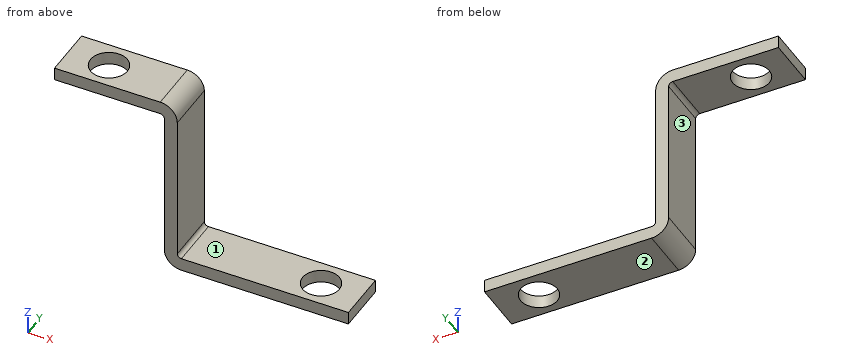
```python
from build123d import *

# Parameters (mm, degrees)
SKETCH1_W                    = 30
SKETCH1_H                    = 12.7
BOSS_EXTRUDE1_DEPTH          = 3.175
EDGE_FLANGE1_STRIP_W         = 14.7
EDGE_FLANGE1_STRIP_H         = 3.175
EDGE_FLANGE1_STRIP_CUT_DEPTH = 12.7
EDGE_FLANGE1_DEPTH           = 12.7
EDGE_FLANGE2_STRIP_W         = 14.7
EDGE_FLANGE2_STRIP_H         = 3.175
EDGE_FLANGE2_STRIP_CUT_DEPTH = 12.7
EDGE_FLANGE2_DEPTH           = 12.7
M8_CLEARANCE_HOLE1_D         = 9


# Sheet-metal steps are written as plain solids
with BuildPart() as part:
    # Sketch1 → Boss-Extrude1 (new body)
    with BuildSketch(Plane.XY):
        with Locations((15, 6.35)):
            Rectangle(SKETCH1_W, SKETCH1_H)
    extrude(amount=BOSS_EXTRUDE1_DEPTH)

    # Edge-Flange1 strip (across the edge) → Edge-Flange1 strip cut (cut)
    with BuildSketch(Plane(origin=(30, 12.7, 0), x_dir=(-1, 0, 0), z_dir=(0, -1, 0))):
        with Locations((-3.175, -1.5875)):
            Rectangle(EDGE_FLANGE1_STRIP_W, EDGE_FLANGE1_STRIP_H)
    extrude(amount=EDGE_FLANGE1_STRIP_CUT_DEPTH, mode=Mode.SUBTRACT)

    # Edge-Flange1 section (across the edge) → Edge-Flange1 (add)
    with BuildSketch(Plane(origin=(30, 12.7, 0), x_dir=(-1, 0, 0), z_dir=(0, -1, 0))):
        with BuildLine():
            Line((0, 1), (0, 41.32))
            Line((0, 41.32), (3.175, 41.32))
            Line((3.175, 41.32), (3.175, 1))
            ThreePointArc((3.175, 1), (3.467893219, 0.292893219), (4.175, 0))
            Line((4.175, 0), (4.175, -3.175))
            ThreePointArc((4.175, -3.175), (1.222829189, -1.952170811), (0, 1))
        make_face()
    extrude(amount=EDGE_FLANGE1_DEPTH)

    # Edge-Flange2 strip (across the edge) → Edge-Flange2 strip cut (cut)
    with BuildSketch(Plane(origin=(30, 0, -41.32), x_dir=(0, 0, 1), z_dir=(0, 1, 0))):
        with Locations((-3.175, -1.5875)):
            Rectangle(EDGE_FLANGE2_STRIP_W, EDGE_FLANGE2_STRIP_H)
    extrude(amount=EDGE_FLANGE2_STRIP_CUT_DEPTH, mode=Mode.SUBTRACT)

    # Edge-Flange2 section (across the edge) → Edge-Flange2 (add)
    with BuildSketch(Plane(origin=(30, 0, -41.32), x_dir=(0, 0, 1), z_dir=(0, 1, 0))):
        with BuildLine():
            Line((0, 1), (0, 41.825))
            Line((0, 41.825), (3.175, 41.825))
            Line((3.175, 41.825), (3.175, 1))
            ThreePointArc((3.175, 1), (3.467893219, 0.292893219), (4.175, 0))
            Line((4.175, 0), (4.175, -3.175))
            ThreePointArc((4.175, -3.175), (1.222829189, -1.952170811), (0, 1))
        make_face()
    extrude(amount=EDGE_FLANGE2_DEPTH)

    # M8 Clearance Hole1 (through all)
    with Locations(Plane(origin=(0, 0, -41.32), x_dir=(-1, 0, 0), z_dir=(0, 0, -1))):
        with Locations((-61.825, 6.35), (-10, 6.35)):
            Hole(M8_CLEARANCE_HOLE1_D / 2)


solid = part.part
```
Check sheet for the modelled part. Datum: model origin and axes. Units: mm. Face numbers are marked on the shaded views. A direction names the side the tool comes from. Give positions to 0.01 mm unless a question says otherwise; leave off trailing zeros. Write each loop counter-clockwise with the first axis right and the second up, starting at its lowest first coordinate (ties: lowest second). Pieces come first, ordered by that corner, then holes. Notation, with made-up numbers: (-3, 60.25) - (16, 60.25) arc R27 cw to (16, 92.25) - close; hole circle Ø9 at (81.5, 42.5). An arc over 180 degrees is marked (long way). Answer as a JSON object with one key per item and string values. Group by question number.
1) Depth check by flat-ended pin: P1, Ø3, axis at x = 28, y = 5.5, coming from the -Z side; P2, Ø6, axis at y = 4, z = -19, coming from the +X side; P3, Ø2, axis at x = 14, y = 6, coming from the -Z side. Enter the tip coordinate at first touch or a pass-through.
2) Sectioned sample at D-D (x = 37). Record the cut outline in (y, z) (3 decimals), then the cut area to 3 significant figures.
3) Sectioned sample at B-B (x = 10). Record the cut outline in (y, z) (3 decimals).
4) Sectioned sample at C-C (z = -7). Record the cut outline in (x, y) (3 decimals).
5) Thickness scan on probe 1 along Y at (x, z) = (10, 1); probe 2 along Z at (x, y) = (5.5, 2.5) (3 decimals); probe 3 along X at (y, z) = (4.75, -6) (3 decimals). Record the ranges inside material, lowest first. Write a range as from..to.
6) Sectioned sample at A-A (y = 6.35). Record the cut outline in (x, z) (3 decimals).
7) Access from +Z, -Z, +X, -X, +Y, -Y to the whole of each face (thin tool, end or side, straight path). Record for the marked faces 1, 2 and 3.
Geometry results:
{
 "1": {"P1": "stops at z = -41.04", "P2": "stops at x = 30", "P3": "stops at z = 0"},
 "2": {"outline": "(0, -41.32) - (12.7, -41.32) - (12.7, -38.145) - (0, -38.145) - close", "area": "40.3 mm^2"},
 "3": {"outline": "(0, 0) - (1.85, 0) - (1.85, 3.175) - (0, 3.175) - close; (10.85, 0) - (12.7, 0) - (12.7, 3.175) - (10.85, 3.175) - close"},
 "4": {"outline": "(26.825, 0) - (30, 0) - (30, 12.7) - (26.825, 12.7) - close"},
 "5": {"probe 1": "y = 0..1.85, 10.85..12.7", "probe 2": "z = 0..3.175", "probe 3": "x = 26.825..30"},
 "6": {"outline": "(0, 0) - (5.5, 0) - (5.5, 3.175) - (0, 3.175) - close; (14.5, 0) - (25.825, 0) arc R1 cw to (26.825, -1) - (26.825, -37.145) arc R4.175 ccw to (31, -41.32) - (57.325, -41.32) - (57.325, -38.145) - (31, -38.145) arc R1 cw to (30, -37.145) - (30, -1) arc R4.175 ccw to (25.825, 3.175) - (14.5, 3.175) - close; (66.325, -41.32) - (71.825, -41.32) - (71.825, -38.145) - (66.325, -38.145) - close"},
 "7": {"face 1": "+Z, +X, +Y, -Y", "face 2": "-Z, +X, -X, +Y, -Y", "face 3": "-Z, -X, +Y, -Y"}
}
